The listing builds one solid part. Answer for the finished solid, in the listing's coordinates (mm). A direction names the side the tool comes from. Round coordinates to 2 decimals unless told otherwise and drop trailing zeros. Order: outer loops, then holes, each group sorted by start corner. A loop starts at its lowest first (then second) coordinate and runs counter-clockwise, first axis right, second up. Notation, with made-up numbers: M 12,88 L 46,88 A18 ccw 46,93 Z; hole C -38,44 d7. An arc over 180 degrees is marked long. Put each result on its own line as item: value. Start each with the question number.
1. Consider line 1 (X direction, y = 7.5, z = 0); line 2 (Z direction, x = 0, y = 8.25); line 3 (X direction, y = 1.6, z = 0) (3 decimals). Determine where each line is inside the solid, lowest interval first.
2. Which of the six approach directions +Z, -Z, +X, -X, +Y, -Y give full straight-line access (tool end or side, diameter ignored) to faces 3 (the face through (0, 0, 0)), 4 (the face through (-3.746, 7.013, 0.165))?
3. The part is cut by section A-A (x = 0). Give the vertices of the cut face in (y, z) (3 decimals), then the cut area to 3 significant figures.
4. The mould has two halves that part along Z. Classify faces 1 (the face through (-3.023, 2.083, -0.097)), 2 (the face through (3, 11.14, -3)): +Z half, -Z half, draft (parallel to the pull), parting line (faces both ways), or undercut.
5. Each of these flat-tipped pins is pushed along its axis until it touches: pin 1 Ø2 at (x, z) = (1.5, 1.5) entering from +Y; pin 2 Ø1.5 at (x, z) = (-1, 0) entering from +Y; pin 3 Ø1.5 at (x, y) = (2, 1.5) entering from -Z. Where does it stop, or does it pass through?
6. The part is cut by section B-B (z = 0). Give the vertices of the cut face in (x, y) (3 decimals).
7. The part is cut by section C-C (z = 4). Give the vertices of the cut face in (x, y).
Autodesk Inventor part; units mm, degrees
ref_plane "YZ Plane" through (0, 0, 0) normal (1, 0, 0) x (0, 1, 0)
ref_plane "XZ Plane" through (0, 0, 0) normal (0, 1, 0) x (-1, 0, 0)
ref_plane "XY Plane" through (0, 0, 0) normal (0, 0, 1) x (1, 0, 0)
sketch "Sketch1" plane through (0, 0, 0) normal (0, 1, 0) x (-1, 0, 0)
  circle A0 centre (0, 0) radius 6
  dimension "d0" = 12
extrude "Extrusion1" add sketch "Sketch1" along normal blind 3
sketch "Sketch2" plane through (0, 3, 0) normal (0, 1, 0) x (1, 0, 0)
  circle A0 centre (0, 0) radius 3.025
  line L0 (1.975, -3) -> (1.975, 3)
  line L1 (-3.025, 0) -> (1.975, 0)
  point P0 (1.975, 2.2913)
  point P1 (1.975, -2.2913)
  dimension "d3" = 6.05
  dimension "d4" = 5
extrude "Extrusion2" cut sketch "Sketch2" against normal blind 1.86 contours L0 L1 A0 | A0 L1 L0
sketch "Sketch4" plane through (0, 3, 0) normal (0, 1, 0) x (1, 0, 0)
  circle A0 centre (0, 0) radius 3.75
  circle A1 centre (0, 0) radius 6
  dimension "d15" = 7.5
  dimension "d16" = 12
extrude "Extrusion4" add sketch "Sketch4" along normal blind 8.14
sketch "Sketch5" plane through (0, 0, 0) normal (0, -1, 0) x (1, 0, 0)
  circle A0 centre (0, 0) radius 6
  circle A1 centre (0, 6) radius 0.4
  dimension "d17" = 0.8
extrude "Extrusion5" cut sketch "Sketch5" against normal through all contours A1 A0 | A0 A1 picked at (-0.0157, 5.8666) picked at (0.014, 6.1316)
pattern_circular "Circular Pattern2" count 30 over 360 about axis through (0, 0, 0) along (0, 1, 0) of "Extrusion5"
properties part number "Knob Rotory Encoder"
Resolved:
1. line 1: -6 to -3.75, 3.75 to 6
1. line 2: -5.6 to -3.75, 3.75 to 5.6
1. line 3: -6 to -3.025, 1.975 to 6
2. face 3: +Z, -Z, +X, -X, -Y
2. face 4: +Y
3. outline: M 0,-5.6 L 11.14,-5.6 L 11.14,-3.75 L 3,-3.75 L 3,-3.025 L 1.14,-3.025 L 1.14,3.025 L 3,3.025 L 3,3.75 L 11.14,3.75 L 11.14,5.6 L 0,5.6 Z
3. area: 52.5 mm2
4. face 1: undercut
4. face 2: draft
5. pin 1: y = 3
5. pin 2: y = 1.14
5. pin 3: z = -5.77
6. outline: M -6,0 L 6,0 L 6,11.14 L 3.75,11.14 L 3.75,3 L 1.975,3 L 1.975,1.14 L -3.025,1.14 L -3.025,3 L -3.75,3 L -3.75,11.14 L -6,11.14 Z
7. outline: M -4.06,0 L 4.06,0 L 4.06,11.14 L -4.06,11.14 Z
